```python
from build123d import *

# Parameters (mm, degrees)
SKETCH1_W                     = 166.5
SKETCH1_H                     = 111
BOSS_EXTRUDE1_DEPTH           = 30.5
SHELL1_T                      = -4.5
CUT_EXTRUDE1_REACH            = 105.377
SKETCH2_W                     = 157
SKETCH2_H                     = 92
TAP_DRILL_FOR_6_32_TAP1_D     = 2.7051
TAP_DRILL_FOR_6_32_TAP1_DEPTH = 4.5
LPATTERN1_COUNT               = 2
LPATTERN1_PITCH               = 30.5
SKETCH7_W                     = 102
SKETCH7_H                     = 4.5
CUT_EXTRUDE2_DEPTH            = 5
CUT_EXTRUDE3_START            = -157
CUT_EXTRUDE3_DEPTH            = 157


with BuildPart() as part:
    # Sketch1 → Boss-Extrude1 (new body)
    with BuildSketch(Plane(origin=(0, 0, 0), x_dir=(1, 0, 0), z_dir=(0, 1, 0))):
        Rectangle(SKETCH1_W, SKETCH1_H)
    extrude(amount=BOSS_EXTRUDE1_DEPTH)

    # Shell1
    shell1_openings = [part.faces().sort_by_distance(p)[0] for p in [
        (0, 30.5, 0),
        (-83.25, 15.25, 0),
    ]]
    offset(amount=SHELL1_T, openings=shell1_openings, kind=Kind.INTERSECTION)

    # Sketch2 → Cut-Extrude1 (cut, up to next)
    with BuildSketch(Plane(origin=(0, 4.5, 0), x_dir=(1, 0, 0), z_dir=(0, 1, 0)), mode=Mode.PRIVATE) as cut_extrude1_sk1:
        with Locations((0.25, 0)):
            Rectangle(SKETCH2_W, SKETCH2_H)
    cut_extrude1_tool1 = extrude(cut_extrude1_sk1.sketch, amount=-CUT_EXTRUDE1_REACH, mode=Mode.PRIVATE) & part.part
    add(cut_extrude1_tool1.solids().sort_by_distance((0.25, 4.5, 0))[0], mode=Mode.SUBTRACT)

    # Tap Drill for #6-32 Tap1
    with Locations(Plane(origin=(0, 0, -55.5), x_dir=(-1, 0, 0), z_dir=(0, 0, -1))):
        with Locations((42.66, 10.84), (-58.75, 10.84)):
            tap_drill_for_6_32_tap1 = Hole(TAP_DRILL_FOR_6_32_TAP1_D / 2, depth=TAP_DRILL_FOR_6_32_TAP1_DEPTH)

    # Mirror1: Tap Drill for #6-32 Tap1 across plane
    add(tap_drill_for_6_32_tap1.mirror(Plane.XY), mode=Mode.SUBTRACT)


with BuildPart() as lpattern1_1:
    # LPattern1: pattern copy
    add(part.part.moved(Location(Vector(0, 1, 0) * (1 * LPATTERN1_PITCH))))


with BuildPart() as part_1:
    add(part.part)

    # Combine1: union LPattern1_1
    add(lpattern1_1.part)

    # Sketch7 → Cut-Extrude2 (cut)
    with BuildSketch(Plane.ZY.offset(83.25)):
        with Locations((0, 32.75)):
            Rectangle(SKETCH7_W, SKETCH7_H)
    extrude(amount=-CUT_EXTRUDE2_DEPTH, mode=Mode.SUBTRACT)

    # Sketch8 → Cut-Extrude3 (cut)
    with BuildSketch(Plane.ZY.offset(78.25).offset(CUT_EXTRUDE3_START)):
        Polygon((-51, 30.5), (-46, 35), (-46, 30.5), align=None)
        Polygon((51, 30.5), (46, 30.5), (46, 35), align=None)
    extrude(amount=CUT_EXTRUDE3_DEPTH, mode=Mode.SUBTRACT)


solid = part_1.part
```
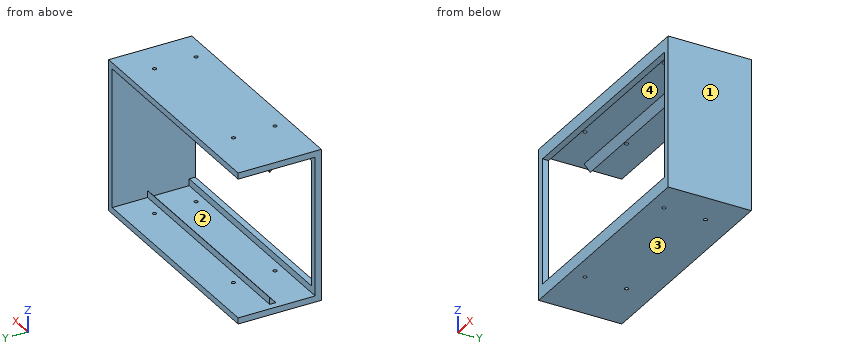
For this review, take the finished solid that the model builds, in its own axes (mm). Face numbers are marked on the shaded views. A direction names the side the tool comes from. Round coordinates to 2 decimals unless told otherwise and drop trailing zeros. Order: outer loops, then holes, each group sorted by start corner. A loop starts at its lowest first (then second) coordinate and runs counter-clockwise, first axis right, second up. Notation, with made-up numbers: (-34, 30) -> (-10, 30) arc R20 ccw to (-10, 52) -> close; hole circle Ø7 at (-0.75, -34.75). An arc over 180 degrees is marked (long way). Use a Markdown table: item, result.
Item 1: Machinability: for the marked faces 1 and 2, which of the approach directions +Z, -Z, +X, -X, +Y, -Y give a long, thin tool a straight path to every point of the face, cutting with its end or side? Answer none if there is none.
Resolved:
| item | result |
|---|---|
| face 1 | +Z, -Z, +X, +Y, -Y |
| face 2 | -X |
Item 2: Take a section at A-A (z = 18.5). State the section outline as (x, y) points.
Resolved:
| item | result |
|---|---|
| outline | (-83.25, 0) -> (-78.25, 0) -> (-78.25, 4.5) -> (-83.25, 4.5) -> close; (78.75, 0) -> (83.25, 0) -> (83.25, 61) -> (78.75, 61) -> close |
Item 3: Take a section at B-B (x = -37.5). State the section outline as (y, z) points.
Resolved:
| item | result |
|---|---|
| outline | (0, -55.5) -> (61, -55.5) -> (61, -51) -> (35, -51) -> (35, -46) -> (30.5, -51) -> (4.5, -51) -> (4.5, -46) -> (0, -46) -> close; (0, 46) -> (4.5, 46) -> (4.5, 51) -> (30.5, 51) -> (35, 46) -> (35, 51) -> (61, 51) -> (61, 55.5) -> (0, 55.5) -> close |
Item 4: For line 1 along Y through (x, z) = (58.75, -53); line 2 along X through (y, z) = (41.34, -52.9); line 3 along Z through (x, y) = (67, 54), list the stretches that pass through material, from the lowest coordinate up. Write a range as [from, to].
Resolved:
| item | result |
|---|---|
| line 1 | y = [0, 9.49], [12.19, 39.99], [42.69, 61] |
| line 2 | x = [-83.25, -44.01], [-41.31, 57.4], [60.1, 83.25] |
| line 3 | z = [-55.5, -51], [51, 55.5] |
Item 5: Draft analysis for pull direction Y (two halves, no side actions). For the marked faces 3 and 4, state which applies: +Y half, -Y half, draft (parallel to the pull), parting line (faces both ways), or undercut.
Resolved:
| item | result |
|---|---|
| face 3 | draft |
| face 4 | undercut |
Item 6: Take a section at C-C (y = 55.5). State the section outline as (x, z) points.
Resolved:
| item | result |
|---|---|
| outline | (-83.25, -55.5) -> (83.25, -55.5) -> (83.25, 55.5) -> (-83.25, 55.5) -> (-83.25, 51) -> (78.75, 51) -> (78.75, -51) -> (-83.25, -51) -> close |
Item 7: For pin 1 (2 mm diameter, centred on y = 32, z = -48, fed in from -X); pin 2 (4.5 mm diameter, centred on x = -42.66, y = 10.84, fed in from -Z); pin 3 (8 mm diameter, centred on y = 51, z = -41.5, fed in from -X); pin 4 (1.5 mm diameter, centred on x = -19.5, z = 47.5, fed in from +Y), all flat-tipped, find the tip position at first contact; note any pin that passes through.
Resolved:
| item | result |
|---|---|
| pin 1 | stops at x = -78.25 |
| pin 2 | stops at z = -55.5 |
| pin 3 | stops at x = 78.75 |
| pin 4 | stops at y = 35 |
